Autodesk Inventor part; units mm, degrees
ref_plane "YZ Plane" through (0, 0, 0) normal (1, 0, 0) x (0, 1, 0)
ref_plane "XZ Plane" through (0, 0, 0) normal (0, 1, 0) x (-1, 0, 0)
ref_plane "XY Plane" through (0, 0, 0) normal (0, 0, 1) x (1, 0, 0)
sketch "Sketch1" plane through (0, 0, 0) normal (1, 0, 0) x (0, 1, 0)
  line L0 (5, -46.5) -> (-5, -46.5)
  line L1 (-5, -46.5) -> (-5, 46.5)
  line L2 (-5, 46.5) -> (5, 46.5)
  line L3 (5, 46.5) -> (5, -46.5)
  line L4 (5, -46.5) -> (-5, 46.5) construction
  line L5 (-5, -46.5) -> (5, 46.5) construction
  circle A0 centre (1.5, 43.5) radius 1
  circle A1 centre (1.5, -42.5) radius 1
  line L6 (-2, 46.5) -> (-2, 5)
  line L7 (-2, 5) -> (-5, 0)
  point P0 (0, 0)
  dimension "d0" = 2
  dimension "d2" = 86
  dimension "d3" = 93
  dimension "d4" = 3.5
  dimension "d5" = 6.5
  dimension "d6" = 4
  dimension "d20" = 3.5
  dimension "d21" = 5
extrude "Extrusion1" add sketch "Sketch1" along normal blind 4.5 contours L0 L1 L7 L6 L2 L3
sketch "Sketch2" plane through (4.5, 0, 0) normal (1, 0, 0) x (0, 0, -1)
  circle A0 centre (-43.5, 1.5) radius 1
  circle A1 centre (-43.5, 1.5) radius 3.25
  circle A2 centre (42.5, 1.5) radius 1
  circle A3 centre (42.5, 1.5) radius 3.25
  point P0 (0, 0)
  dimension "d9" = 6.5
extrude "Extrusion2" add sketch "Sketch2" against normal blind 23
fillet "Fillet1" radius 1 3 edges at (0, -1.6869, 42.8626) (0, 4.6869, 42.8626) (0, 1.5, -39.25)
chamfer "Chamfer1" distance 0.5 angle 45 6 edges at (4.5, 0.7929, 44.2071) (4.5, 2.2071, 42.7929) (4.5, 2.2071, -43.2071) (4.5, 0.7929, -41.7929) (-18.5, 1.5, -41.5) (-18.5, 1.5, 44.5)
properties part number "PCB_support"
Source: CAD feature listing. Evaluate the final solid. Frame: model axes, mm. A direction names the side the tool comes from. Round coordinates to 2 decimals unless told otherwise and drop trailing zeros. Loops run counter-clockwise (first coordinate to the right, second up) from the corner with the lowest first, then second, coordinate; pieces in that order, holes last. Notation, with made-up numbers: M 50,85.5 L 80,85.5 A17 cw 80,89.5 Z; hole C 61.5,61 d10. An arc over 180 degrees is marked long. Put each result on its own line as item: value.
(1) Section A-A, the plane x = 2. Return loops of the section in (y, z), and give its area (3 significant figures).
Solutions:
outline: M -5,-46.5 L 5,-46.5 L 5,46.5 L 2.75,46.5 A3.25 ccw 0.25,46.5 L -2,46.5 L -2,5 L -5,0 Z; hole C 1.5,-42.5 d2; hole C 1.5,43.5 d2
area: 792 mm²
(2) Access query for faces 5 (the face through (2, -2, 26)), 6 (the face through (0, 4.4, -46)), 7 (the face through (-9.628, 0.255, -45.502)), 8 (the face through (2, 4, 46.5)). Directions: +Z, -Z, +X, -X, +Y, -Y. A direction counts if a zero-diameter tool reaches every point of the face in a straight line with its end or side. Return the directions, or none.
Solutions:
face 5: +Z, +X, -X, -Y
face 6: -Z, -X, +Y
face 7: -X
face 8: +Z, +X, -X, +Y
(3) Section C-C, the plane y = 1.5. Return loops of the section in (x, z).
Solutions:
outline: M -18.5,-45.75 L -1,-45.75 A1 cw -0.03,-46.5 L 4.5,-46.5 L 4.5,-44 L 4,-43.5 L -18,-43.5 L -18.5,-44 Z; M -18.5,-41 L -18,-41.5 L 4,-41.5 L 4.5,-41 L 4.5,42 L 4,42.5 L -18,42.5 L -18.5,42 L -18.5,40.25 L -1,40.25 A1 cw 0,39.25 L 0,-38.25 A1 cw -1,-39.25 L -18.5,-39.25 Z; M -18.5,45 L -18,44.5 L 4,44.5 L 4.5,45 L 4.5,46.75 L -18.5,46.75 Z
(4) First-contact query: pin 1 (1.5 mm diameter, centred on y = -3.5, z = 37, fed in from -X); pin 2 (1.3 mm diameter, centred on y = 4.5, z = -46, fed in from -X); pin 3 (2.5 mm diameter, centred on y = 1.5, z = 43.5, fed in from -X); pin 4 (0.7 mm diameter, centred on x = 0.5, y = 3.5, fed in from +Z). Flat tips, straight axial feed; report the tip coordinate or a pass-through.
Solutions:
pin 1: through
pin 2: x = -0.04
pin 3: x = -18.25
pin 4: z = 46.5
(5) Section B-B, the plane z = -42.5. Return loops of the section in (x, y).
Solutions:
outline: M -18.5,-1.75 L -1,-1.75 A1 cw 0,-2.75 L 0,-5 L 4.5,-5 L 4.5,0 L 4,0.5 L -18,0.5 L -18.5,0 Z; M -18.5,3 L -18,2.5 L 4,2.5 L 4.5,3 L 4.5,5 L -0.34,5 A1 cw -1,4.75 L -18.5,4.75 Z
(6) Section D-D, the plane x = -11.5. Return loops of the section in (y, z), and give its area (3 significant figures).
Solutions:
outline: C 1.5,-42.5 d6.5; C 1.5,43.5 d6.5; hole C 1.5,-42.5 d2; hole C 1.5,43.5 d2
area: 60.1 mm²
(7) Ray query, line 1 (Y direction, x = -5, z = 43.5); line 2 (Z direction, x = -3.75, y = 2); line 3 (X direction, y = 2.5, z = 26). Return the intervals inside material, ascending. Write a range as [from, to].
Solutions:
line 1: [-1.75, 0.5], [2.5, 4.75]
line 2: [-45.71, -43.37], [-41.63, -39.29], [40.29, 42.63], [44.37, 46.71]
line 3: [0, 4.5]
(8) Pull-direction query (Z, two-part tool) for faces 1 (the face through (-9.395, 1.643, 46.747)), 2 (the face through (2, -1, 46.5)), 3 (the face through (-18.5, 0.8, 45)), 4 (the face through (0, 0, -2)); classes: released by +Z, released by -Z, zero draft, split by the parting line, or undercut.
Solutions:
face 1: undercut
face 2: released by +Z
face 3: zero draft
face 4: undercut
